Verification items for the finished model (mm, model axes). A direction names the side the tool comes from. Coordinates: 2 decimals unless noted, no trailing zeros. Loops run counter-clockwise (first coordinate to the right, second up) from the corner with the lowest first, then second, coordinate; pieces in that order, holes last. Notation, with made-up numbers: (70.5, -5) - (127.5, -5) arc R7 cw to (127.5, 8) - close; hole circle Ø7 at (82.5, 22). An arc over 180 degrees is marked (long way). Answer as CSV lines item,"result". Start each with the question number.
1. Cross-section at D-D (y = 81.5). Enter the section's corners in (x, z).
2. Gauge pin test, flat ends, axial feed: P1, Ø10, axis at x = 4.5, y = 57, coming from the +Z side; P2, Ø4, axis at y = 11.5, z = -5.5, coming from the +X side; P3, Ø1.4, axis at y = 60.5, z = 10.5, coming from the +X side; P4, Ø10, axis at x = 6.5, z = 1.5, coming from the -Y side. Record the tip position at first contact, or that the pin passes through.
3. Cross-section at C-C (z = 0). Enter the section's corners in (x, y), plus the area to 3 significant figures.
4. Release check for a two-part mould opening along Z. For faces 1 (the cylindrical face through (-0.46, -3.29, 3.52)), 2 (the cylindrical face through (0, 73.5, -10.8)), 3 (the cylindrical face through (-2.222, 43.575, 10.006)) record: pulls with the +Z half, pulls with the -Z half, needs draft (parallel to the pull), parting line crosses it, or undercut.
5. Cross-section at B-B (x = 0). Enter the section's corners in (y, z), plus the area to 3 significant figures.
6. Material ranges on line 1 (X direction, y = 45, z = 0); line 2 (Y direction, x = -5.25, z = 7), recorded low to high. Write a range as [from, to].
7. Cross-section at A-A (y = 61). Enter the section's corners in (x, z), plus the area to 3 significant figures.
8. Set-up check for faces 4 (the flat face through (0, 1.35, 0)), 5 (the flat face through (0, 0, -5)), 6 (the cylindrical face through (0, 50.5, 10.8)), 7 (the cylindrical face through (-2.493, 43.144, 11.227)): record each of +Z, -Z, +X, -X, +Y, -Y from which the full face is reachable in a straight line by a thin tool's end or side.
```python
from build123d import *

# Parameters (mm, degrees)
SKETCH1_R               = 11.5
SKETCH1_R_2             = 10.25
BOSS_EXTRUDE1_DEPTH     = 87
SKETCH2_R               = 10.25
BOSS_EXTRUDE2_DEPTH     = 1.35
SKETCH3_R               = 3.55
BOSS_EXTRUDE3_DEPTH     = 6.66
CUT_EXTRUDE1_DEPTH      = 12.5
CUT_EXTRUDE1_DEPTH_BACK = 12.5
FILLET1_R               = 0.5


with BuildPart() as part:
    # Sketch1 → Boss-Extrude1 (new body)
    with BuildSketch(Plane(origin=(0, 0, 0), x_dir=(1, 0, 0), z_dir=(0, 1, 0))):
        Circle(SKETCH1_R)
        Circle(SKETCH1_R_2, mode=Mode.SUBTRACT)
    extrude(amount=BOSS_EXTRUDE1_DEPTH)

    # Sketch2 → Boss-Extrude2 (add)
    with BuildSketch(Plane.XZ):
        Circle(SKETCH2_R)
    extrude(amount=-BOSS_EXTRUDE2_DEPTH)

    # Sketch3 → Boss-Extrude3 (add)
    with BuildSketch(Plane.XZ):
        Circle(SKETCH3_R)
    extrude(amount=BOSS_EXTRUDE3_DEPTH)

    # Sketch4 → Cut-Extrude1 (cut, two sides)
    with BuildSketch(Plane.XY) as cut_extrude1_sk:
        with BuildLine():
            Line((-2, 71.5), (-2, 52.5))
            ThreePointArc((-2, 52.5), (0, 50.5), (2, 52.5))
            Line((2, 52.5), (2, 71.5))
            ThreePointArc((2, 71.5), (0, 73.5), (-2, 71.5))
        make_face()
    extrude(amount=CUT_EXTRUDE1_DEPTH, mode=Mode.SUBTRACT)
    extrude(cut_extrude1_sk.sketch, amount=-CUT_EXTRUDE1_DEPTH_BACK, mode=Mode.SUBTRACT)

    # Fillet1
    fillet1_edges = [part.edges().sort_by_distance(p)[0] for p in [
        (-3.55, 0, 0),
        (-3.55, -6.66, 0),
        (-11.5, 0, 0),
    ]]
    fillet(fillet1_edges, radius=FILLET1_R)


solid = part.part
```
Values follow:
1,outline,"circle Ø23 at (0, 0); hole circle Ø20.5 at (0, 0)"
2,P1,"stops at z = 11.32"
2,P2,"stops at x = 10.95"
2,P3,"stops at x = 6.02"
2,P4,"stops at y = -6.66"
3,outline,"(-11.5, 0.5) arc R0.5 ccw to (-11, 0) - (-4.05, 0) arc R0.5 cw to (-3.55, -0.5) - (-3.55, -6.16) arc R0.5 ccw to (-3.05, -6.66) - (3.05, -6.66) arc R0.5 ccw to (3.55, -6.16) - (3.55, -0.5) arc R0.5 cw to (4.05, 0) - (11, 0) arc R0.5 ccw to (11.5, 0.5) - (11.5, 87) - (10.25, 87) - (10.25, 1.35) - (-10.25, 1.35) - (-10.25, 87) - (-11.5, 87) - close"
3,area,"292 mm²"
4,face 1,"parting line crosses it"
4,face 2,"needs draft"
4,face 3,"undercut"
5,outline,"(-6.66, -3.05) arc R0.5 ccw to (-6.16, -3.55) - (-0.5, -3.55) arc R0.5 cw to (0, -4.05) - (0, -11) arc R0.5 ccw to (0.5, -11.5) - (50.5, -11.5) - (50.5, -10.25) - (1.35, -10.25) - (1.35, 10.25) - (50.5, 10.25) - (50.5, 11.5) - (0.5, 11.5) arc R0.5 ccw to (0, 11) - (0, 4.05) arc R0.5 cw to (-0.5, 3.55) - (-6.16, 3.55) arc R0.5 ccw to (-6.66, 3.05) - close; (73.5, -11.5) - (87, -11.5) - (87, -10.25) - (73.5, -10.25) - close; (73.5, 10.25) - (87, 10.25) - (87, 11.5) - (73.5, 11.5) - close"
5,area,"235 mm²"
6,line 1,"x = [-11.5, -10.25], [10.25, 11.5]"
6,line 2,"y = [0, 1.35]"
7,outline,"(-2, -11.32) - (-2, -10.05) arc R10.25 cw to (-2, 10.05) - (-2, 11.32) arc R11.5 ccw to start; (2, -11.32) arc R11.5 ccw to (2, 11.32) - (2, 10.05) arc R10.25 cw to (2, -10.05) - close"
7,area,"75.4 mm²"
8,face 4,"+Y"
8,face 5,"-Y"
8,face 6,"+Z, -Z"
8,face 7,"+Y, -Y"
